```python
from build123d import *

# Parameters (mm, degrees)
BOSS_EXTRUDE1_DEPTH = 6.5
CUT_EXTRUDE3_DEPTH  = 71.600991494
SKETCH4_W           = 4
SKETCH4_H           = 58
SKETCH4_W_2         = 1.7
SKETCH4_H_2         = 65
CUT_EXTRUDE4_DEPTH  = 4.5
SKETCH5_R           = 1.25
BOSS_EXTRUDE2_DEPTH = 2
SKETCH6_R           = 1.25
CUT_EXTRUDE5_DEPTH  = 2


with BuildPart() as part:
    # Sketch1 → Boss-Extrude1 (new body)
    with BuildSketch(Plane(origin=(0, 0, 0), x_dir=(1, 0, 0), z_dir=(0, 1, 0))):
        Polygon((1.5, -32.5), (6.5, -32.5), (6.5, 32.5), (1.5, 32.5), (1.5, 35), (-5.5, 35), (-5.5, 32.5), (-1.5, 32.5), (-1.5, -32.5), (-5.5, -32.5), (-5.5, -35), (1.5, -35), align=None)
    extrude(amount=-BOSS_EXTRUDE1_DEPTH)

    # Sketch3 → Cut-Extrude3 (cut, through all)
    with BuildSketch(Plane.XY.offset(35)):
        with BuildLine():
            Line((-5.5, 0), (-5.5, -3.25))
            ThreePointArc((-5.5, -3.25), (-4.548097039, -0.951902961), (-2.25, 0))
            Line((-2.25, 0), (-5.5, 0))
        make_face()
        with BuildLine():
            Line((-5.5, -6.5), (-2.25, -6.5))
            ThreePointArc((-2.25, -6.5), (-4.548097039, -5.548097039), (-5.5, -3.25))
            Line((-5.5, -3.25), (-5.5, -6.5))
        make_face()
    extrude(amount=-CUT_EXTRUDE3_DEPTH, mode=Mode.SUBTRACT)

    # Sketch4 → Cut-Extrude4 (cut)
    with BuildSketch(Plane.XZ.offset(6.5)):
        with Locations((4.5, 0)):
            Rectangle(SKETCH4_W, SKETCH4_H)
        with Locations((-0.65, 0)):
            Rectangle(SKETCH4_W_2, SKETCH4_H_2)
    extrude(amount=-CUT_EXTRUDE4_DEPTH, mode=Mode.SUBTRACT)

    # Sketch5 → Boss-Extrude2 (add)
    with BuildSketch(Plane.XY.offset(-32.5)):
        with Locations((-3.25, -3.25)):
            Circle(SKETCH5_R)
    boss_extrude2 = extrude(amount=BOSS_EXTRUDE2_DEPTH)

    # Sketch6 → Cut-Extrude5 (cut)
    with BuildSketch(Plane(origin=(0, 0, -32.5), x_dir=(-1, 0, 0), z_dir=(0, 0, -1))):
        with Locations((-4.75, -3.25)):
            Circle(SKETCH6_R)
    cut_extrude5 = extrude(amount=-CUT_EXTRUDE5_DEPTH, mode=Mode.SUBTRACT)

    # Mirror1: Boss-Extrude2, Cut-Extrude5 across plane
    add(boss_extrude2.mirror(Plane.XY))
    add(cut_extrude5.mirror(Plane.XY), mode=Mode.SUBTRACT)


solid = part.part
```
Geometry check sheet. Reference: the model listing, model coordinates, mm. A direction names the side the tool comes from. Give positions to 0.01 mm unless a question says otherwise; leave off trailing zeros. Write each loop counter-clockwise with the first axis right and the second up, starting at its lowest first coordinate (ties: lowest second). Pieces come first, ordered by that corner, then holes. Notation, with made-up numbers: (76.5, -10.75) - (116.5, -10.75) arc R16 cw to (116.5, 8.25) - close; hole circle Ø7 at (-37.5, 19). An arc over 180 degrees is marked (long way). Use a Markdown table: item, result.
Q1. Go/stop test with flat-tipped pins: P1, Ø2.5, axis at x = 3.5, y = -3, coming from the +Z side; P2, Ø1.2, axis at y = -2, z = -33.5, coming from the +X side; P3, Ø2, axis at x = -3, z = -1.5, coming from the -Y side; P4, Ø3, axis at x = 5, y = -3.5, coming from the -Z side. Record where each tip stops, or that it passes through.
Computed:
| item | result |
|---|---|
| P1 | stops at z = 32.5 |
| P2 | stops at x = 1.5 |
| P3 | passes through |
| P4 | stops at z = -32.5 |
Q2. Section check A-A, the plane z = 23.5. Enter the section's corners in (x, y).
Computed:
| item | result |
|---|---|
| outline | (-1.5, -2) - (0.2, -2) - (0.2, -6.5) - (2.5, -6.5) - (2.5, -2) - (6.5, -2) - (6.5, 0) - (-1.5, 0) - close |
Q3. Section check C-C, the plane y = -1. Enter the section's corners in (x, z).
Computed:
| item | result |
|---|---|
| outline | (-4.6, -35) - (1.5, -35) - (1.5, -32.5) - (6.5, -32.5) - (6.5, 32.5) - (1.5, 32.5) - (1.5, 35) - (-4.6, 35) - (-4.6, 32.5) - (-1.5, 32.5) - (-1.5, -32.5) - (-4.6, -32.5) - close |
Q4. Set-up check for faces 4 (the face through (3, -3, -32.5)), 5 (the face through (4, -2, 0)), 6 (the face through (-3, -3, 30.5)), 7 (the face through (3, -3, 32.5)), 8 (the face through (-2.06, -2.87, 31.51)): record each of +Z, -Z, +X, -X, +Y, -Y from which the full face is reachable in a straight line by a thin tool's end or side.
Computed:
| item | result |
|---|---|
| face 4 | -Z, +X, +Y, -Y |
| face 5 | +X, -Y |
| face 6 | -X, +Y, -Y |
| face 7 | +Z, +X, +Y, -Y |
| face 8 | none |
Q5. Thickness scan on L1, parallel to Y at x = 4.75, z = -32.05; L2, parallel to Z at x = -1.25, y = -4; L3, parallel to Z at x = -3.5, y = -2.75. Record the ranges inside material, lowest first. Write a range as [from, to].
Computed:
| item | result |
|---|---|
| L1 | y = [-6.5, -4.5], [-2, 0] |
| L2 | z = [-35, -32.5], [32.5, 35] |
| L3 | z = [-35, -30.5], [30.5, 35] |
Q6. Section check D-D, the plane x = -3.25. Enter the section's corners in (y, z).
Computed:
| item | result |
|---|---|
| outline | (-6.34, -35) - (-0.16, -35) - (-0.16, -32.5) - (-2, -32.5) - (-2, -30.5) - (-4.5, -30.5) - (-4.5, -32.5) - (-6.34, -32.5) - close; (-6.34, 32.5) - (-4.5, 32.5) - (-4.5, 30.5) - (-2, 30.5) - (-2, 32.5) - (-0.16, 32.5) - (-0.16, 35) - (-6.34, 35) - close |
Q7. Draft check along Y on faces 1 (the face through (4, -4, 29)), 2 (the face through (2, 0, 0)), 3 (the face through (6, -3.2, 31.5)). Enter one of: pulls with the +Y half, pulls with the -Y half, needs draft (parallel to the pull), parting line crosses it, or undercut.
Computed:
| item | result |
|---|---|
| face 1 | needs draft |
| face 2 | pulls with the +Y half |
| face 3 | undercut |
Q8. Section check B-B, the plane x = 4.75. Enter the section's corners in (y, z).
Computed:
| item | result |
|---|---|
| outline | (-6.5, -32.5) - (-4.5, -32.5) - (-4.5, -30.5) - (-2, -30.5) - (-2, -32.5) - (0, -32.5) - (0, 32.5) - (-2, 32.5) - (-2, 30.5) - (-4.5, 30.5) - (-4.5, 32.5) - (-6.5, 32.5) - (-6.5, 29) - (-2, 29) - (-2, -29) - (-6.5, -29) - close |
